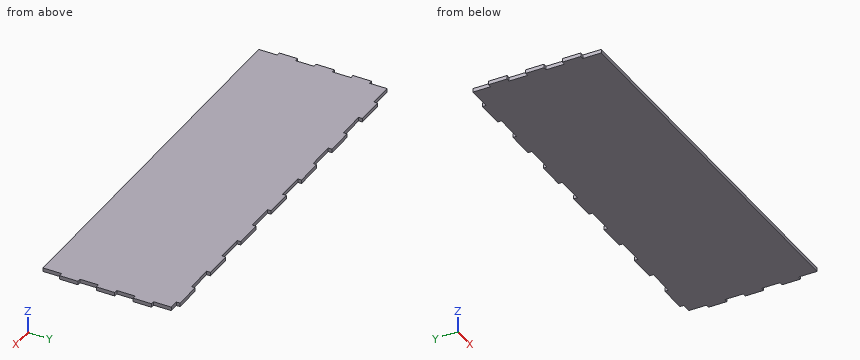
```python
from build123d import *

# Parameters (mm, degrees)
SKETCH1_W               = 275.57984
SKETCH1_H               = 90.8685
BOSS_EXTRUDE1_DEPTH     = 2.54
SKETCH2_W               = 2.54
SKETCH2_H               = 12.7
CUT_EXTRUDE1_DEPTH      = 146.109561114
LPATTERN1_COUNT         = 4
LPATTERN1_PITCH         = 25.4
MIRROR1_COPY_1_SKETCH_W = 2.54
MIRROR1_COPY_1_SKETCH_H = 12.7
MIRROR1_COPY_1_DEPTH    = 146.109561114
MIRROR1_COPY_2_SKETCH_W = 2.54
MIRROR1_COPY_2_SKETCH_H = 12.7
MIRROR1_COPY_2_DEPTH    = 146.109561114
MIRROR1_COPY_3_SKETCH_W = 2.54
MIRROR1_COPY_3_SKETCH_H = 12.7
MIRROR1_COPY_3_DEPTH    = 146.109561114
SKETCH3_W               = 19.05
SKETCH3_H               = 2.54
CUT_EXTRUDE2_DEPTH      = 146.109561114
LPATTERN2_COUNT         = 8
LPATTERN2_PITCH         = 38.1


with BuildPart() as part:
    # Sketch1 → Boss-Extrude1 (new body)
    with BuildSketch(Plane.XY):
        Rectangle(SKETCH1_W, SKETCH1_H)
    extrude(amount=BOSS_EXTRUDE1_DEPTH)

    # Sketch2 → Cut-Extrude1 (cut, through all)
    with BuildSketch(Plane.XY.offset(2.54)):
        with Locations((136.51992, -39.08425)):
            Rectangle(SKETCH2_W, SKETCH2_H)
    cut_extrude1 = extrude(amount=-CUT_EXTRUDE1_DEPTH, mode=Mode.SUBTRACT)

    # LPattern1: Cut-Extrude1 ×4
    with Locations(*[(0, i * LPATTERN1_PITCH, 0) for i in range(1, LPATTERN1_COUNT)]):
        add(cut_extrude1, mode=Mode.SUBTRACT)

    # Mirror1: Cut-Extrude1 across plane
    add(cut_extrude1.mirror(Plane(origin=(0, 0, 0), x_dir=(0, 0, 1), z_dir=(1, 0, 0))), mode=Mode.SUBTRACT)

    # Mirror1 copy 1 sketch → Mirror1 copy 1 (cut, through all)
    with BuildSketch(Plane(origin=(0, 25.4, 2.54), x_dir=(-1, 0, 0), z_dir=(0, 0, 1))):
        with Locations((136.51992, 39.08425)):
            Rectangle(MIRROR1_COPY_1_SKETCH_W, MIRROR1_COPY_1_SKETCH_H)
    extrude(amount=-MIRROR1_COPY_1_DEPTH, mode=Mode.SUBTRACT)

    # Mirror1 copy 2 sketch → Mirror1 copy 2 (cut, through all)
    with BuildSketch(Plane(origin=(0, 50.8, 2.54), x_dir=(-1, 0, 0), z_dir=(0, 0, 1))):
        with Locations((136.51992, 39.08425)):
            Rectangle(MIRROR1_COPY_2_SKETCH_W, MIRROR1_COPY_2_SKETCH_H)
    extrude(amount=-MIRROR1_COPY_2_DEPTH, mode=Mode.SUBTRACT)

    # Mirror1 copy 3 sketch → Mirror1 copy 3 (cut, through all)
    with BuildSketch(Plane(origin=(0, 76.2, 2.54), x_dir=(-1, 0, 0), z_dir=(0, 0, 1))):
        with Locations((136.51992, 39.08425)):
            Rectangle(MIRROR1_COPY_3_SKETCH_W, MIRROR1_COPY_3_SKETCH_H)
    extrude(amount=-MIRROR1_COPY_3_DEPTH, mode=Mode.SUBTRACT)

    # Sketch3 → Cut-Extrude2 (cut, through all)
    with BuildSketch(Plane.XY.offset(2.54)):
        with Locations((-128.26492, 44.16425)):
            Rectangle(SKETCH3_W, SKETCH3_H)
    cut_extrude2 = extrude(amount=-CUT_EXTRUDE2_DEPTH, mode=Mode.SUBTRACT)

    # LPattern2: Cut-Extrude2 ×8
    with Locations(*[(i * LPATTERN2_PITCH, 0, 0) for i in range(1, LPATTERN2_COUNT)]):
        add(cut_extrude2, mode=Mode.SUBTRACT)


solid = part.part
```
Read the model definition and answer for the solid it produces. Units are mm, in the model's axes. Coordinates: 2 decimals unless noted, no trailing zeros. Order: outer loops, then holes, each group sorted by start corner. A loop starts at its lowest first (then second) coordinate and runs counter-clockwise, first axis right, second up. Notation, with made-up numbers: (-32.75, -1.5) - (0.25, -1.5) arc R25 cw to (0.25, 20.5) - close; hole circle Ø1 at (11, 44.5). An arc over 180 degrees is marked (long way). Answer as a JSON object with one key per item and string values. Group by question number.
Item 1: Consider probe 1 along Y at (x, z) = (-10.5, 1.85); probe 2 along X at (y, z) = (13.5, 1.4). Determine where each line is inside the solid, lowest interval first. Write a range as from..to.
Item 2: Section B-B (y = 35) is taken. Give the vertices of the cut face in (x, z).
Item 3: Flat-ended cylindrical pins translate along their axes: P1, Ø1.3, axis at y = 44, z = 1.5, coming from the +X side; P2, Ø1, axis at y = -19, z = 1.5, coming from the -X side; P3, Ø0.8, axis at x = 137, z = 1.5, coming from the -Y side. Find the tip coordinate at first contact, or state that the pin passes through.
Item 4: Section A-A (x = 99.5) is taken. Give the vertices of the cut face in (y, z), plus the area to 3 significant figures.
Results are:
{
 "1": {"probe 1": "y = -45.43..42.89", "probe 2": "x = -135.25..135.25"},
 "2": {"outline": "(-135.25, 0) - (135.25, 0) - (135.25, 2.54) - (-135.25, 2.54) - close"},
 "3": {"P1": "stops at x = 128.91", "P2": "stops at x = -135.25", "P3": "stops at y = -32.73"},
 "4": {"outline": "(-45.43, 0) - (42.89, 0) - (42.89, 2.54) - (-45.43, 2.54) - close", "area": "224 mm^2"}
}
